Check sheet for the drawn part. Datum: minimum x, y, z corner. Units: mm. Coordinates: 2 decimals unless noted, no trailing zeros. Order: outer loops, then holes, each group sorted by start corner. A loop starts at its lowest first (then second) coordinate and runs counter-clockwise, first axis right, second up.
Q1. Thickness scan on line 1 (X direction, y = 8, z = 0.9); line 2 (X direction, y = 31, z = 3.45); line 3 (Y direction, x = 18.5, z = 3.2). Record the ranges inside material, lowest first.
Q2. Depth check by flat-ended pin: P1, Ø1.6, axis at x = 7.32, y = 7.32, coming from the +Z side; P2, Ø1.5, axis at y = 44.5, z = 2, coming from the +X side. Enter the tip coordinate at first touch or a pass-through.
Q3. Cross-section at A-A, the plane y = 25. Record the boundary of the cut face in (x, z).
Q4. Cross-section at D-D, the plane y = 32.5. Record the boundary of the cut face in (x, z) (1 decimal).
Q5. Draft check along Y on the marked faces 1, 2, 3 and 4. Enter one of: pulls with the +Y half, pulls with the -Y half, needs draft (parallel to the pull), parting line crosses it, or undercut.
Q6. Cross-section at C-C, the plane z = 2.95. Count the separate pieces of the cut face and the enclosed holes in it, and give its area (3 significant figures).
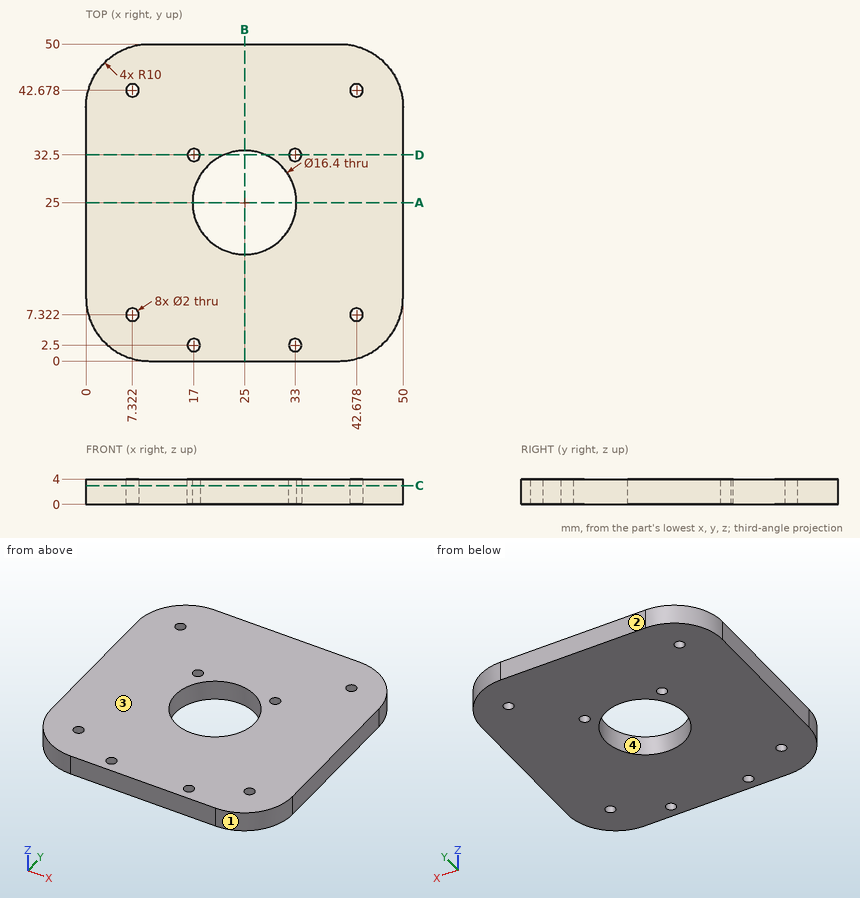
Check values:
1. line 1: x = 0.2 to 6.59, 8.06 to 41.94, 43.41 to 49.8
1. line 2: x = 0 to 19.41, 30.59 to 50
1. line 3: y = 0 to 20, 30 to 50
2. P1: passes through
2. P2: stops at x = 49.27
3. outline: (0, 0) - (16.8, 0) - (16.8, 4) - (0, 4) - close; (33.2, 0) - (50, 0) - (50, 4) - (33.2, 4) - close
4. outline: (0, 0) - (16, 0) - (16, 4) - (0, 4) - close; (18, 0) - (21.7, 0) - (21.7, 4) - (18, 4) - close; (28.3, 0) - (32, 0) - (32, 4) - (28.3, 4) - close; (34, 0) - (50, 0) - (50, 4) - (34, 4) - close
5. face 1: pulls with the -Y half
5. face 2: pulls with the +Y half
5. face 3: needs draft
5. face 4: undercut
6. separate pieces: 1
6. enclosed holes: 9
6. area: 2,180 mm2
